Design review of the part built by this model. Coordinates are the model's own, in mm. Round coordinates to 2 decimals unless told otherwise and drop trailing zeros. Loops run counter-clockwise (first coordinate to the right, second up) from the corner with the lowest first, then second, coordinate; pieces in that order, holes last. Notation, with made-up numbers: (-8.75, -35.5) -> (-2.75, -35.5) arc R16 cw to (-2.75, -12.5) -> close; hole circle Ø1 at (26, 8.25). An arc over 180 degrees is marked (long way). Use a Markdown table: item, result. Add a question column.
Autodesk Inventor part; units mm, degrees
ref_plane "YZ Plane" through (0, 0, 0) normal (1, 0, 0) x (0, 1, 0)
ref_plane "XZ Plane" through (0, 0, 0) normal (0, 1, 0) x (-1, 0, 0)
ref_plane "XY Plane" through (0, 0, 0) normal (0, 0, 1) x (1, 0, 0)
sketch "スケッチ1" plane through (0, 0, 0) normal (0, 0, 1) x (1, 0, 0)
  line L0 (-80, -38.5) -> (80, -38.5)
  line L1 (80, -38.5) -> (80, 38.5)
  line L2 (80, 38.5) -> (-80, 38.5)
  line L3 (-80, 38.5) -> (-80, -38.5)
  line L4 (-80, -38.5) -> (80, 38.5) construction
  line L5 (80, -38.5) -> (-80, 38.5) construction
  point P0 (0, 0)
  dimension "d0" = 160
  dimension "d1" = 77
extrude "プレート1" add sketch "スケッチ1" along normal blind 1
sketch "スケッチ2" plane through (0, 0, 1) normal (0, 0, 1) x (1, 0, 0)
  line L0 (-80, -38.5) -> (-80, 38.5)
  line L1 (80, -38.5) -> (-80, -38.5)
  line L2 (80, 38.5) -> (80, -38.5)
  line L3 (-80, 38.5) -> (80, 38.5)
  line L4 (75, 33.5) -> (75, -33.5)
  line L5 (75, -33.5) -> (-75, -33.5)
  line L6 (-75, -33.5) -> (-75, 33.5)
  line L7 (-75, 33.5) -> (75, 33.5)
  point P0 (0, 0)
  dimension "d3" = 5
hole "穴1" at (-75, 33.5, 1) at (-75, -33.5, 1) at (75, -33.5, 1) at (75, 33.5, 1) direction (0, 0, -1) diameter 3.2 depth 1
sketch "スケッチ3" plane through (0, 0, 1) normal (0, 0, 1) x (1, 0, 0)
  line L0 (80, -38.5) -> (-80, -38.5)
  point P0 (0, 0)
  point P1 (-60, -13.5)
  point P2 (60, -13.5)
  dimension "d11" = 60
  dimension "d12" = 60
  dimension "d13" = 25
  dimension "d14" = 25
hole "穴2" at (-60, -13.5, 1) at (60, -13.5, 1) direction (0, 0, -1) diameter 5.3 end through all
equation "\"d9\" = Thickness"
equation "\"d20\" = Thickness"
equation "\"d2\" = Thickness"
equation "\"BendRadius\" = Thickness"
equation "\"BendReliefWidth\" = Thickness"
equation "\"BendReliefDepth\" = 0.5 * Thickness"
equation "\"CornerReliefSize\" = 4 * Thickness"
equation "\"MinimumRemnant\" = 2 * Thickness"
equation "\"TransitionRadius\" = BendRadius"
equation "\"JacobiRadiusSize\" = Thickness"
equation "\"GapSize\" = Thickness"
properties part number "plate4" material "CFRP"
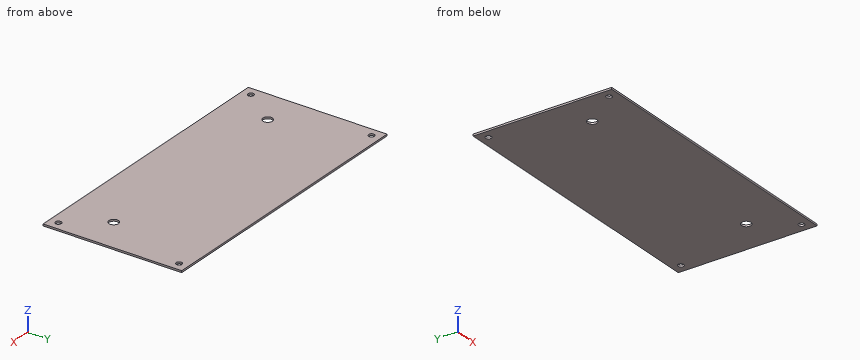
1. Consider section A-A on y = -33.5. State the section outline as (x, z) points.
2. To check wall thickness, follow probe 1 along Y at (x, z) = (-75, 0.3); probe 2 along X at (y, z) = (-33.5, 0.6); probe 3 along X at (y, z) = (-13.5, 0.6). State the ranges of each line that lie inside material, in increasing order. Write a range as from..to.
3. Consider section B-B on x = -75. State the section outline as (y, z) points, plus the area to 3 significant figures.
4. Consider section C-C on x = 60. State the section outline as (y, z) points, plus the area to 3 significant figures.
Verdict:
| question | item | result |
|---|---|---|
| 1 | outline | (-80, 0) -> (-76.6, 0) -> (-76.6, 1) -> (-80, 1) -> close; (-73.4, 0) -> (73.4, 0) -> (73.4, 1) -> (-73.4, 1) -> close; (76.6, 0) -> (80, 0) -> (80, 1) -> (76.6, 1) -> close |
| 2 | probe 1 | y = -38.5..-35.1, -31.9..31.9, 35.1..38.5 |
| 2 | probe 2 | x = -80..-76.6, -73.4..73.4, 76.6..80 |
| 2 | probe 3 | x = -80..-62.65, -57.35..57.35, 62.65..80 |
| 3 | outline | (-38.5, 0) -> (-35.1, 0) -> (-35.1, 1) -> (-38.5, 1) -> close; (-31.9, 0) -> (31.9, 0) -> (31.9, 1) -> (-31.9, 1) -> close; (35.1, 0) -> (38.5, 0) -> (38.5, 1) -> (35.1, 1) -> close |
| 3 | area | 70.6 mm² |
| 4 | outline | (-38.5, 0) -> (-16.15, 0) -> (-16.15, 1) -> (-38.5, 1) -> close; (-10.85, 0) -> (38.5, 0) -> (38.5, 1) -> (-10.85, 1) -> close |
| 4 | area | 71.7 mm² |
